```python
from build123d import *

# Parameters (mm, degrees)
BOSS_EXTRUDE1_DEPTH    = 6.35
F_10_32_TAPPED_HOLE2_D = 4.0386
FILLET2_R              = 12.7
CUT_EXTRUDE3_DEPTH     = 89.032651707
FILLET3_DEPTH          = 6.35
SKETCH12_R             = 14.3129
CUT_EXTRUDE4_DEPTH     = 89.032651707
SKETCH13_R             = 2.0193
CUT_EXTRUDE5_DEPTH     = 89.032651707


with BuildPart() as part:
    # Sketch1 → Boss-Extrude1 (new body)
    with BuildSketch(Plane(origin=(0, 0, 0), x_dir=(1, 0, 0), z_dir=(0, 1, 0))):
        Polygon((59.54395, 22.225), (84.94395, 22.225), (84.94395, -22.225), (59.54395, -22.225), (-59.54395, -22.225), (-59.54395, 22.225), align=None)
    extrude(amount=BOSS_EXTRUDE1_DEPTH)

    # #10-32 Tapped Hole2 (through all)
    with Locations(Plane(origin=(0, 6.35, 0), x_dir=(1, 0, 0), z_dir=(0, 1, 0))):
        with Locations((-46.84395, 9.525), (-21.44395, 9.525), (-21.44395, -9.525), (-46.84395, -9.525)):
            Hole(F_10_32_TAPPED_HOLE2_D / 2)

    # Fillet2
    fillet2_edges = [part.edges().sort_by_distance(p)[0] for p in [
        (-59.54395, 3.175, 22.225),
        (-59.54395, 3.175, -22.225),
    ]]
    fillet(fillet2_edges, radius=FILLET2_R)

    # Sketch11 → Cut-Extrude3 (cut, through all)
    with BuildSketch(Plane(origin=(0, 6.35, 0), x_dir=(1, 0, 0), z_dir=(0, 1, 0))):
        with BuildLine():
            Line((-46.84395, 15.875), (-21.44395, 15.875))
            ThreePointArc((-21.44395, 15.875), (-27.353773893, 11.848032834), (-25.767954708, 4.874679228))
            Line((-25.767954708, 4.874679228), (-34.14395, 1.697847323))
            Line((-34.14395, 1.697847323), (-42.519945292, 4.874679228))
            ThreePointArc((-42.519945292, 4.874679228), (-40.934126107, 11.848032834), (-46.84395, 15.875))
        make_face()
        with BuildLine():
            Line((-15.09395, -9.525), (-15.09395, 9.525))
            ThreePointArc((-15.09395, 9.525), (-16.90021853, 5.089123048), (-21.291431679, 3.176831905))
            Line((-21.291431679, 3.176831905), (-29.667426971, 0))
            Line((-29.667426971, 0), (-21.291431679, -3.176831905))
            ThreePointArc((-21.291431679, -3.176831905), (-16.90021853, -5.089123048), (-15.09395, -9.525))
        make_face()
        with BuildLine():
            Line((-53.19395, 9.525), (-53.19395, -9.525))
            ThreePointArc((-53.19395, -9.525), (-51.38768147, -5.089123048), (-46.996468321, -3.176831905))
            Line((-46.996468321, -3.176831905), (-38.620473029, 0))
            Line((-38.620473029, 0), (-46.996468321, 3.176831905))
            ThreePointArc((-46.996468321, 3.176831905), (-51.38768147, 5.089123048), (-53.19395, 9.525))
        make_face()
        with BuildLine():
            Line((-46.84395, -15.875), (-21.44395, -15.875))
            ThreePointArc((-21.44395, -15.875), (-27.353773893, -11.848032834), (-25.767954708, -4.874679228))
            Line((-25.767954708, -4.874679228), (-34.14395, -1.697847323))
            Line((-34.14395, -1.697847323), (-42.519945292, -4.874679228))
            ThreePointArc((-42.519945292, -4.874679228), (-40.934126107, -11.848032834), (-46.84395, -15.875))
        make_face()
    extrude(amount=-CUT_EXTRUDE3_DEPTH, mode=Mode.SUBTRACT)

    # Fillet3: read off the stored shape, not the designer's step
    # Fillet3 outline → Fillet3 (add)
    with BuildSketch(Plane(origin=(0, 0, 0), x_dir=(1, 0, 0), z_dir=(0, 1, 0))):
        with BuildLine():
            ThreePointArc((-18.722521429, 3.787724817), (-16.276262891, 3.63950655), (-15.09395, 1.492814743))
            Line((-15.09395, 1.492814743), (-15.09395, 9.525))
            ThreePointArc((-15.09395, 9.525), (-16.077220482, 6.130782227), (-18.722521429, 3.787724817))
        make_face()
        with BuildLine():
            Line((-15.09395, -9.525), (-15.09395, -1.492814743))
            ThreePointArc((-15.09395, -1.492814743), (-16.276262891, -3.63950655), (-18.722521429, -3.787724817))
            ThreePointArc((-18.722521429, -3.787724817), (-16.077220482, -6.130782227), (-15.09395, -9.525))
        make_face()
        with BuildLine():
            ThreePointArc((-21.662369003, 3.036143487), (-21.315105323, 3.140185377), (-20.956567225, 3.19373172))
            ThreePointArc((-20.956567225, 3.19373172), (-21.12388789, 3.183071252), (-21.291431679, 3.176831905))
            Line((-21.291431679, 3.176831905), (-21.662369003, 3.036143487))
        make_face()
        with BuildLine():
            ThreePointArc((-21.291431679, -3.176831905), (-21.12388789, -3.183071252), (-20.956567225, -3.19373172))
            ThreePointArc((-20.956567225, -3.19373172), (-21.315105323, -3.140185377), (-21.662369003, -3.036143487))
            Line((-21.662369003, -3.036143487), (-21.291431679, -3.176831905))
        make_face()
        with BuildLine():
            ThreePointArc((-23.405745013, -2.374919079), (-25.044990125, 0), (-23.405745013, 2.374919079))
            Line((-23.405745013, 2.374919079), (-29.667426971, 0))
            Line((-29.667426971, 0), (-23.405745013, -2.374919079))
        make_face()
        with BuildLine():
            ThreePointArc((-41.106674817, 12.246428571), (-40.95845655, 14.692687109), (-38.811764743, 15.875))
            Line((-38.811764743, 15.875), (-46.84395, 15.875))
            ThreePointArc((-46.84395, 15.875), (-43.449732228, 14.891729517), (-41.106674817, 12.246428571))
        make_face()
        with BuildLine():
            Line((-21.44395, 15.875), (-29.476135257, 15.875))
            ThreePointArc((-29.476135257, 15.875), (-27.32944345, 14.692687109), (-27.181225183, 12.246428571))
            ThreePointArc((-27.181225183, 12.246428571), (-24.838167772, 14.891729517), (-21.44395, 15.875))
        make_face()
        with BuildLine():
            ThreePointArc((-39.533862913, 3.742123461), (-40.965188005, 5.110562055), (-40.979062875, 7.090744671))
            ThreePointArc((-40.979062875, 7.090744671), (-41.630398839, 5.899895272), (-42.519945292, 4.874679228))
            Line((-42.519945292, 4.874679228), (-39.533862913, 3.742123461))
        make_face()
        with BuildLine():
            ThreePointArc((-25.767954708, 4.874679228), (-26.657501161, 5.899895272), (-27.308837125, 7.090744671))
            ThreePointArc((-27.308837125, 7.090744671), (-27.322711995, 5.110562055), (-28.754037087, 3.742123461))
            Line((-28.754037087, 3.742123461), (-25.767954708, 4.874679228))
        make_face()
        with BuildLine():
            ThreePointArc((-33.243195112, 2.03948396), (-34.14395, 1.874403039), (-35.044704888, 2.03948396))
            Line((-35.044704888, 2.03948396), (-34.14395, 1.697847323))
            Line((-34.14395, 1.697847323), (-33.243195112, 2.03948396))
        make_face()
        with BuildLine():
            Line((-38.620473029, 0), (-44.882154987, 2.374919079))
            ThreePointArc((-44.882154987, 2.374919079), (-43.242909875, 0), (-44.882154987, -2.374919079))
            Line((-44.882154987, -2.374919079), (-38.620473029, 0))
        make_face()
        with BuildLine():
            ThreePointArc((-47.331332775, 3.19373172), (-46.972794677, 3.140185377), (-46.625530997, 3.036143487))
            Line((-46.625530997, 3.036143487), (-46.996468321, 3.176831905))
            ThreePointArc((-46.996468321, 3.176831905), (-47.16401211, 3.183071252), (-47.331332775, 3.19373172))
        make_face()
        with BuildLine():
            Line((-46.996468321, -3.176831905), (-46.625530997, -3.036143487))
            ThreePointArc((-46.625530997, -3.036143487), (-46.972794677, -3.140185377), (-47.331332775, -3.19373172))
            ThreePointArc((-47.331332775, -3.19373172), (-47.16401211, -3.183071252), (-46.996468321, -3.176831905))
        make_face()
        with BuildLine():
            ThreePointArc((-53.19395, 1.492814743), (-52.011637109, 3.63950655), (-49.565378571, 3.787724817))
            ThreePointArc((-49.565378571, 3.787724817), (-52.210679518, 6.130782227), (-53.19395, 9.525))
            Line((-53.19395, 9.525), (-53.19395, 1.492814743))
        make_face()
        with BuildLine():
            ThreePointArc((-53.19395, -9.525), (-52.210679518, -6.130782227), (-49.565378571, -3.787724816))
            ThreePointArc((-49.565378571, -3.787724816), (-52.011637109, -3.63950655), (-53.19395, -1.492814743))
            Line((-53.19395, -1.492814743), (-53.19395, -9.525))
        make_face()
        with BuildLine():
            ThreePointArc((-40.979062875, -7.090744671), (-40.965188005, -5.110562055), (-39.533862913, -3.742123461))
            Line((-39.533862913, -3.742123461), (-42.519945292, -4.874679228))
            ThreePointArc((-42.519945292, -4.874679228), (-41.630398839, -5.899895272), (-40.979062875, -7.090744671))
        make_face()
        with BuildLine():
            Line((-34.14395, -1.697847323), (-35.044704888, -2.03948396))
            ThreePointArc((-35.044704888, -2.03948396), (-34.14395, -1.874403039), (-33.243195112, -2.03948396))
            Line((-33.243195112, -2.03948396), (-34.14395, -1.697847323))
        make_face()
        with BuildLine():
            ThreePointArc((-38.811764743, -15.875), (-40.95845655, -14.692687109), (-41.106674817, -12.246428571))
            ThreePointArc((-41.106674817, -12.246428571), (-43.449732228, -14.891729517), (-46.84395, -15.875))
            Line((-46.84395, -15.875), (-38.811764743, -15.875))
        make_face()
        with BuildLine():
            Line((-25.767954708, -4.874679228), (-28.754037087, -3.742123461))
            ThreePointArc((-28.754037087, -3.742123461), (-27.322711995, -5.110562055), (-27.308837125, -7.090744671))
            ThreePointArc((-27.308837125, -7.090744671), (-26.657501161, -5.899895272), (-25.767954708, -4.874679228))
        make_face()
        with BuildLine():
            ThreePointArc((-27.181225183, -12.246428571), (-27.32944345, -14.692687109), (-29.476135257, -15.875))
            Line((-29.476135257, -15.875), (-21.44395, -15.875))
            ThreePointArc((-21.44395, -15.875), (-24.838167772, -14.891729517), (-27.181225183, -12.246428571))
        make_face()
    extrude(amount=FILLET3_DEPTH)

    # Sketch12 → Cut-Extrude4 (cut, through all)
    with BuildSketch(Plane(origin=(0, 6.35, 0), x_dir=(1, 0, 0), z_dir=(0, 1, 0))):
        with Locations(Location((62.71895, 2.175, 0), (0, 0, 270))):
            Circle(SKETCH12_R)
    extrude(amount=-CUT_EXTRUDE4_DEPTH, mode=Mode.SUBTRACT)

    # Sketch13 → Cut-Extrude5 (cut, through all)
    with BuildSketch(Plane(origin=(0, 6.35, 0), x_dir=(1, 0, 0), z_dir=(0, 1, 0))):
        with Locations(Location((78.59395, 14.875, 0), (0, 0, 270))):
            Circle(SKETCH13_R)
        with Locations(Location((46.84395, 14.875, 0), (0, 0, 270))):
            Circle(SKETCH13_R)
        with Locations(Location((46.84395, -16.875, 0), (0, 0, 270))):
            Circle(SKETCH13_R)
        with Locations(Location((78.59395, -16.875, 0), (0, 0, 270))):
            Circle(SKETCH13_R)
    extrude(amount=-CUT_EXTRUDE5_DEPTH, mode=Mode.SUBTRACT)


solid = part.part
```
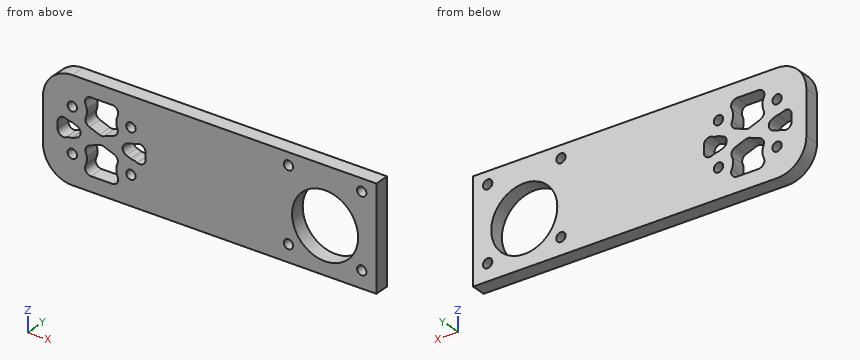
Input: part model. Units: mm. Frame: model coordinates. Coordinates: 2 decimals unless noted, no trailing zeros. Write each loop counter-clockwise with the first axis right and the second up, starting at its lowest first coordinate (ties: lowest second). Pieces come first, ordered by that corner, then holes.
1) Section D-D on z = -19. Output: boundary loops of the cut face in (x, y).
2) Pin query (flat end, axial travel): pin 1 Ø4.5 at (x, z) = (-21.44, 9.52) entering from -Y. Return the tip coordinate at first contact, or that it passes through.
3) Material intervals for line 1 along X through (y, z) = (4, -15); line 2 along Z through (x, y) = (-47.5, 2.5); line 3 along X through (y, z) = (2, -6.5), sorted ascending.
4) Section A-A on x = 72. Output: boundary loops of the cut face in (y, z) (3 decimals).
5) Section B-B on x = -16.5. Output: boundary loops of the cut face in (y, z) (3 decimals), and give its area (3 significant figures).
6) Section C-C on y = 2.75. State how many separate pieces and enclosed holes the cut face has, and give its area (3 significant figures).
Check result:
1. outline: (-55.3, 0) - (84.94, 0) - (84.94, 6.35) - (-55.3, 6.35) - close
2. pin 1: stops at y = 0
3. line 1: x = -58.3 to -40.73, -27.56 to 44.83, 48.86 to 56.36, 69.07 to 76.58, 80.61 to 84.94
3. line 2: z = -22.21 to -11.43, -7.62 to -3.21, 3.21 to 7.62, 11.43 to 22.21
3. line 3: x = -59.54 to -41.14, -27.14 to 49.08, 76.36 to 84.94
4. outline: (0, -22.225) - (6.35, -22.225) - (6.35, -13.071) - (0, -13.071) - close; (0, 8.721) - (6.35, 8.721) - (6.35, 22.225) - (0, 22.225) - close
5. outline: (0, -22.225) - (6.35, -22.225) - (6.35, -3.766) - (0, -3.766) - close; (0, 3.766) - (6.35, 3.766) - (6.35, 22.225) - (0, 22.225) - close
5. area: 234 mm2
6. separate pieces: 1
6. enclosed holes: 13
6. area: 5,140 mm2
